```python
from build123d import *

# Parameters (mm, degrees)
F1_DEPTH = 2


with BuildPart() as f1:
    # F0 (on Top) → F1 (new body)
    with BuildSketch(Plane.XY):
        with BuildLine():
            ThreePointArc((0, 2), (0.585786, 0.585786), (2, 0))
            Line((2, 0), (21, 0))
            ThreePointArc((21, 0), (22.414214, 0.585786), (23, 2))
            Line((23, 2), (23, 16))
            ThreePointArc((23, 16), (22.414214, 17.414214), (21, 18))
            Line((21, 18), (2, 18))
            ThreePointArc((2, 18), (0.585786, 17.414214), (0, 16))
            Line((0, 16), (0, 2))
        make_face()
        with BuildLine():
            Line((5, 6), (5, 9))
            Line((5, 9), (5, 12))
            ThreePointArc((5, 12), (5.585786, 13.414214), (7, 14))
            Line((7, 14), (16, 14))
            ThreePointArc((16, 14), (17.414214, 13.414214), (18, 12))
            Line((18, 12), (18, 9))
            Line((18, 9), (18, 6))
            ThreePointArc((18, 6), (17.414214, 4.585786), (16, 4))
            Line((16, 4), (7, 4))
            ThreePointArc((7, 4), (5.585786, 4.585786), (5, 6))
        make_face(mode=Mode.SUBTRACT)
    extrude(amount=F1_DEPTH)


solid = f1.part
```
Source: CAD feature listing. Evaluate the final solid. Frame: model axes, mm. A direction names the side the tool comes from. Round coordinates to 2 decimals unless told otherwise and drop trailing zeros. Order: outer loops, then holes, each group sorted by start corner. A loop starts at its lowest first (then second) coordinate and runs counter-clockwise, first axis right, second up. Notation, with made-up numbers: (5.5, -34) -> (18.5, -34) arc R26 cw to (18.5, -20) -> close; hole circle Ø7 at (62, 64). An arc over 180 degrees is marked (long way). One line per item, written item: value. Start each with the question number.
Q1. Section query A-A (y = 9.25). Return the cut outline in (x, z).
Q2. Section query C-C (z = 1.6). Return the cut outline in (x, y).
Q3. Draft query along Y for faces 3 (the flat face through (12, 18, 1)), 4 (the flat face through (0, 9, 1)), 5 (the flat face through (5, 9, 1)). Return one class per face: pulls with the +Y half, pulls with the -Y half, needs draft (parallel to the pull), parting line crosses it, or undercut.
Q4. Material intervals for probe 1 along Y at (x, z) = (10.75, 0.2); probe 2 along X at (y, z) = (7.5, 1.2); probe 3 along Y at (x, z) = (17.25, 0.65), sorted ascending.
Q5. Section query B-B (x = 9.25). Return the cut outline in (y, z), plus the area to 3 significant figures.
Q6. Access query for faces 1 (the cylindrical face through (5.6, 4.57, 0.99)), 2 (the flat face through (11, 0, 1)). Directions: +Z, -Z, +X, -X, +Y, -Y. A direction counts if a zero-diameter tool reaches every point of the face in a straight line with its end or side. Return the directions, or none.
Findings below:
1. outline: (0, 0) -> (5, 0) -> (5, 2) -> (0, 2) -> close; (18, 0) -> (23, 0) -> (23, 2) -> (18, 2) -> close
2. outline: (0, 2) arc R2 ccw to (2, 0) -> (21, 0) arc R2 ccw to (23, 2) -> (23, 16) arc R2 ccw to (21, 18) -> (2, 18) arc R2 ccw to (0, 16) -> close; hole (5, 6) arc R2 ccw to (7, 4) -> (16, 4) arc R2 ccw to (18, 6) -> (18, 12) arc R2 ccw to (16, 14) -> (7, 14) arc R2 ccw to (5, 12) -> close
3. face 3: pulls with the +Y half
3. face 4: needs draft
3. face 5: undercut
4. probe 1: 0 to 4, 14 to 18
4. probe 2: 0 to 5, 18 to 23
4. probe 3: 0 to 4.44, 13.56 to 18
5. outline: (0, 0) -> (4, 0) -> (4, 2) -> (0, 2) -> close; (14, 0) -> (18, 0) -> (18, 2) -> (14, 2) -> close
5. area: 16.0 mm²
6. face 1: +Z, -Z
6. face 2: +Z, -Z, +X, -X, -Y
